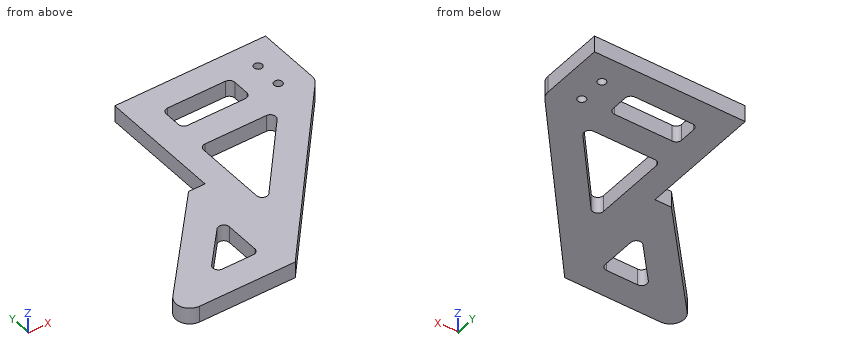
from build123d import *

# Parameters (mm, degrees)
BOSS_EXTRUDE1_DEPTH     = 6
SKETCH4_R               = 1.5
SKETCH4_W               = 25
SKETCH4_H               = 10
CUT_EXTRUDE2_DEPTH      = 1
CUT_EXTRUDE2_DEPTH_BACK = 7
FILLET1_R               = 2
FILLET2_R               = 2
FILLET3_R               = 5


with BuildPart() as part:
    # Sketch1 → Boss-Extrude1 (new body)
    with BuildSketch(Plane.XY):
        Polygon((0, 0), (55, 0), (55, -25), (0, -90), (-46, -90), (-6, -45), (0, -45), align=None)
    extrude(amount=BOSS_EXTRUDE1_DEPTH)

    # Sketch4 → Cut-Extrude2 (cut, two sides)
    with BuildSketch(Plane.XY.offset(6)) as cut_extrude2_sk:
        with Locations((45, -20)):
            Circle(SKETCH4_R)
        with Locations((45, -10)):
            Circle(SKETCH4_R)
        Polygon((9, -30), (9, -63.882376031), (37.669702795, -30), align=None)
        Polygon((-6, -60.051993223), (-23.731561579, -80), (-6, -80), align=None)
        with Locations((22.5, -15)):
            Rectangle(SKETCH4_W, SKETCH4_H)
    extrude(amount=CUT_EXTRUDE2_DEPTH, mode=Mode.SUBTRACT)
    extrude(cut_extrude2_sk.sketch, amount=-CUT_EXTRUDE2_DEPTH_BACK, mode=Mode.SUBTRACT)

    # Fillet1
    fillet1_edges = [part.edges().sort_by_distance(p)[0] for p in [
        (-6, -60.051993223, 3),
        (-6, -80, 3),
        (-23.731561579, -80, 3),
        (10, -20, 3),
        (10, -10, 3),
        (35, -10, 3),
        (35, -20, 3),
    ]]
    fillet(fillet1_edges, radius=FILLET1_R)

    # Fillet2
    fillet2_edges = [part.edges().sort_by_distance(p)[0] for p in [
        (9, -30, 3),
        (37.669702795, -30, 3),
        (9, -63.882376031, 3),
    ]]
    fillet(fillet2_edges, radius=FILLET2_R)

    # Fillet3
    fillet3_edges = [part.edges().sort_by_distance(p)[0] for p in [
        (55, -25, 3),
        (-46, -90, 3),
    ]]
    fillet(fillet3_edges, radius=FILLET3_R)


solid = part.part
Geometry check sheet. Reference: the model listing, model coordinates, mm. Coordinates: 2 decimals unless noted, no trailing zeros. Loops run counter-clockwise (first coordinate to the right, second up) from the corner with the lowest first, then second, coordinate; pieces in that order, holes last. Notation, with made-up numbers: (-16, -15.5) - (17, -15.5) arc R28 cw to (17, 3.5) - close; hole circle Ø11 at (63, 56). An arc over 180 degrees is marked (long way). Use one line per item in the form item = value. Start each with the question number.
Item 1: Thickness scan on probe 1 along Y at (x, z) = (45, 4.1); probe 2 along X at (y, z) = (-35, 3.2); probe 3 along X at (y, z) = (-20.5, 3.4). Record the ranges inside material, lowest first.
Item 2: Section check A-A, the plane z = 1.4. Give the number of separate pieces and of enclosed holes in the cut face, and give its area (3 significant figures).
Item 3: Section check B-B, the plane y = -67. Enter the section's corners in (x, z).
Item 4: Section check D-D, the plane x = 29.5. Enter the section's corners in (y, z), and give its area (3 significant figures).
Item 5: Section check C-C, the plane x = 45. Enter the section's corners in (y, z), and give its area (3 significant figures).
Item 6: Gauge pin test, flat ends, axial feed: pin 1 (1.8 mm diameter, centred on y = -15, z = 4, fed in from -X); pin 2 (3 mm diameter, centred on y = -74.5, z = 3.5, fed in from -X); pin 3 (1.8 mm diameter, centred on x = -1.5, z = 4.5, fed in from +Y). Record the tip position at first contact, or that the pin passes through.
Computed:
q1.probe_1 = -36.82 to -21.5, -18.5 to -11.5, -8.5 to 0
q1.probe_2 = 0 to 9, 33.44 to 46.54
q1.probe_3 = 0 to 43.59, 46.41 to 55
q2.separate_pieces = 1
q2.enclosed_holes = 5
q2.area = 3,400 mm2
q3.outline = (-25.56, 0) - (-12.18, 0) - (-12.18, 6) - (-25.56, 6) - close; (-6, 0) - (19.46, 0) - (19.46, 6) - (-6, 6) - close
q4.outline = (-55.14, 0) - (-39.66, 0) - (-39.66, 6) - (-55.14, 6) - close; (-30, 0) - (-20, 0) - (-20, 6) - (-30, 6) - close; (-10, 0) - (0, 0) - (0, 6) - (-10, 6) - close
q4.area = 213 mm2
q5.outline = (-36.82, 0) - (-21.5, 0) - (-21.5, 6) - (-36.82, 6) - close; (-18.5, 0) - (-11.5, 0) - (-11.5, 6) - (-18.5, 6) - close; (-8.5, 0) - (0, 0) - (0, 6) - (-8.5, 6) - close
q5.area = 185 mm2
q6.pin_1 = 0
q6.pin_2 = -33.56
q6.pin_3 = -45
